Autodesk Inventor part; units mm, degrees
ref_plane "YZ Plane" through (0, 0, 0) normal (1, 0, 0) x (0, 1, 0)
ref_plane "XZ Plane" through (0, 0, 0) normal (0, 1, 0) x (-1, 0, 0)
ref_plane "XY Plane" through (0, 0, 0) normal (0, 0, 1) x (1, 0, 0)
sketch "Sketch2" plane through (0, 0, 0) normal (1, 0, 0) x (0, 1, 0)
  line L0 (11, -16) -> (-11, -16)
  line L1 (-11, -16) -> (-11, 16)
  line L2 (-11, 16) -> (11, 16)
  line L3 (11, 16) -> (11, -16)
  line L4 (11, -16) -> (-11, 16) construction
  line L5 (-11, -16) -> (11, 16) construction
  circle A0 centre (0, -6.5) radius 4.8
  circle A1 centre (0, 6.5) radius 4.8
  line L6 (0, 6.5) -> (0, 0)
  point P0 (0, 0)
  dimension "d8" = 22
  dimension "d9" = 32
  dimension "d14" = 9.6
  dimension "d15" = 13
  dimension "d23" = 6.5
  dimension "d24" = 9.6
  dimension "d25" = 13
extrude "Extrusion2" add sketch "Sketch2" against normal blind 10
shell "Shell1" thickness 2 removed faces 3 at (-10, 8.8868, -1.7838) at (-6.6667, 4.7378, -7.27) at (-6.6667, 4.7378, 5.73)
sketch "Sketch4" plane through (0, 0, 0) normal (0, 1, 0) x (-1, 0, 0)
  line L0 (2, -14) -> (2, 14)
  line L1 (2, 0) -> (4.75, 0) construction
  line L2 (4.75, -11.3497) -> (6.75, -11.3497)
  line L3 (6.75, -11.3497) -> (6.75, 11.3497)
  line L4 (6.75, 11.3497) -> (4.75, 11.3497)
  line L5 (4.75, 11.3497) -> (4.75, -11.3497)
  point P0 (0, 0)
  dimension "d19" = 2.75
  dimension "d20" = 2
extrude "Extrusion4" cut sketch "Sketch4" along normal mid plane 22
sketch "Sketch5" plane through (0, -11, -16) normal (0, -1, 0) x (1, 0, 0)
  line L0 (-10, 2) -> (-10, 30)
  line L1 (-8, 17.5) -> (-10, 17.5)
  line L2 (-10, 17.5) -> (-10, 14.5)
  line L3 (-10, 14.5) -> (-8, 14.5)
  line L4 (-8, 14.5) -> (-8, 17.5)
  line L5 (-8, 17.5) -> (-10, 14.5) construction
  line L6 (-10, 17.5) -> (-8, 14.5) construction
  line L7 (-10, 0) -> (-10, 32)
  point P0 (0, 16)
  dimension "d27" = 3
  dimension "d30" = 2
extrude "Extrusion5" cut sketch "Sketch5" against normal blind 2
sketch "Sketch6" plane through (-2, -9, 14) normal (-1, 0, 0) x (0, 0, 1)
  line L0 (0, 18) -> (0, 0)
  line L1 (-28, 16) -> (0, 16)
  line L2 (0, 16) -> (0, 2)
  line L3 (0, 2) -> (-28, 2)
  line L4 (-28, 2) -> (-28, 16)
  line L5 (-28, 16) -> (0, 2) construction
  line L6 (0, 16) -> (-28, 2) construction
  line L7 (-28, 18) -> (0, 18)
  line L8 (0, 18) -> (0, 0)
  line L9 (0, 0) -> (-28, 0)
  line L10 (-28, 0) -> (-28, 18)
  line L11 (-28, 18) -> (0, 0) construction
  line L12 (0, 18) -> (-28, 0) construction
  point P0 (-14, 9)
  dimension "d31" = 14
extrude "Extrusion6" add sketch "Sketch6" along normal blind 2.75 contours L0 L1 L10 L7 | L0 L9 L10 L3
properties part number "snapConnector_3DPrint"
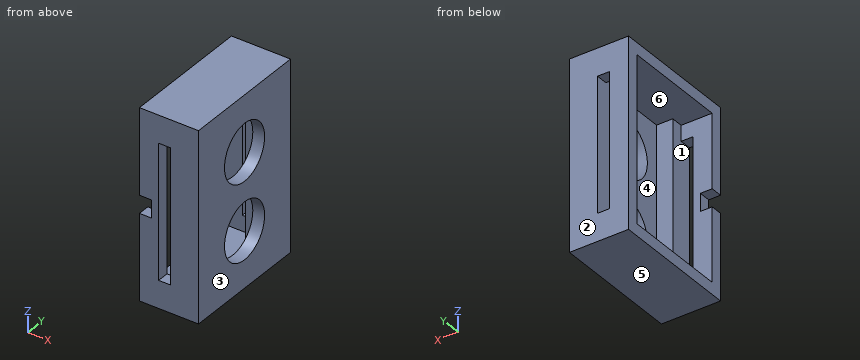
Work out the finished part from the listing and answer in its coordinate system (mm). Face numbers are marked on the shaded views. A direction names the side the tool comes from. Round coordinates to 2 decimals unless told otherwise and drop trailing zeros. Loops run counter-clockwise (first coordinate to the right, second up) from the corner with the lowest first, then second, coordinate; pieces in that order, holes last. Notation, with made-up numbers: M 75.5,11 L 86.5,11 A17 ccw 86.5,39 Z; hole C -2.5,85.25 d9. An arc over 180 degrees is marked long. One line per question, with ' | ' between items. Start each with the question number.
(1) A cutting plane is placed at B-B on y = -4.25. Write down the section's boundary in (x, z), plus the area to 3 significant figures.
(2) A cutting plane is placed at A-A on z = -6.5. Write down the section's boundary in (x, y).
(3) Find the intervals of material crossed by line 1 (Z direction, x = -1.35, y = 0); line 2 (Z direction, x = -5, y = -9.5); line 3 (Y direction, x = -7.5, z = 13.5), in increasing order.
(4) Flat-ended cylindrical pins translate along their axes: pin 1 Ø1.6 at (y, z) = (-9.5, 0) entering from -X; pin 2 Ø8 at (y, z) = (-6.5, 3) entering from +X. Find the tip coordinate at first contact, or state that the pin passes through.
(5) A cutting plane is placed at D-D on x = -4.25. Write down the section's boundary in (y, z).
(6) For a pull along X with two mould halves and no side action, classify the marked faces 1, 2, 3 and 4 as released by +X, released by -X, zero draft, split by the parting line, or undercut.
(7) A cutting plane is placed at C-C on z = 0. Write down the section's boundary in (x, y).
(8) A tool of negligible diameter and unlimited length cuts with its end or side. For the marked faces 5 and 6, from which of +Z, -Z, +X, -X, +Y, -Y can it reach the whole face along a straight path? Write none if from no direction.
Geometry check:
1) outline: M -10,-16 L 0,-16 L 0,-8.73 L -2,-8.73 L -2,-14 L -10,-14 Z; M -10,14 L -2,14 L -2,8.73 L 0,8.73 L 0,16 L -10,16 Z; M -2,-4.27 L 0,-4.27 L 0,4.27 L -2,4.27 Z | area: 78.2 mm²
2) outline: M -10,-11 L -6.75,-11 L -6.75,-9 L -10,-9 Z; M -10,9 L -6.75,9 L -6.75,11 L -10,11 Z; M -4.75,-11 L 0,-11 L 0,-4.8 L -2,-4.8 L -2,-7 L -4.75,-7 Z; M -4.75,7 L -2,7 L -2,4.8 L 0,4.8 L 0,11 L -4.75,11 Z
3) line 1: z = -16 to -11.3, -1.7 to 1.7, 11.3 to 16 | line 2: z = -16 to -11.35, 11.35 to 16 | line 3: y = -11 to -9, 9 to 11
4) pin 1: stops at x = -8 | pin 2: stops at x = 0
5) outline: M -11,-16 L 11,-16 L 11,16 L -11,16 Z; hole M -7,-14 L 7,-14 L 7,14 L -7,14 Z
6) face 1: undercut | face 2: zero draft | face 3: released by +X | face 4: released by -X
7) outline: M -10,9 L -6.75,9 L -6.75,11 L -10,11 Z; M -8,-11 L -6.75,-11 L -6.75,-9 L -8,-9 Z; M -4.75,-11 L 0,-11 L 0,11 L -4.75,11 L -4.75,7 L -2,7 L -2,-7 L -4.75,-7 Z
8) face 5: -Z, +X, -X, +Y, -Y | face 6: -X
